from build123d import *

# Parameters (mm, degrees)
ESTRUSIONE_ESTRUSIONE1_DEPTH = 140
FORO_6_5_6_5_1_D             = 6.5
FORO_6_5_6_5_2_D             = 6.5
FORO_6_5_6_5_2_DEPTH         = 5
FORO_6_5_6_5_2_TIP           = 1.952797012
TAGLIO_ESTRUSIONE3_REACH     = 158.844
SCHIZZO10_R                  = 7
TAGLIO_ESTRUSIONE6_REACH     = 158.844
SMUSSO1_SIZE                 = 3
M3_TAPPED_HOLE1_D            = 2.5
M3_TAPPED_HOLE2_D            = 2.5


with BuildPart() as part:
    # Schizzo1 → Estrusione-Estrusione1 (new body)
    with BuildSketch(Plane.XY):
        Polygon((0, 0), (0, 50), (5, 50), (5, 5), (50, 5), (50, 0), align=None)
    extrude(amount=ESTRUSIONE_ESTRUSIONE1_DEPTH)

    # Foro Ø6.5 (6.5)-1 (through all)
    with Locations(Plane(origin=(0, 0, 0), x_dir=(-1, 0, 0), z_dir=(0, -1, 0))):
        with Locations((-17, -132), (-42, -132)):
            foro_6_5_6_5_1 = Hole(FORO_6_5_6_5_1_D / 2)

    # Foro Ø6.5 (6.5)-2
    with Locations(Plane.ZY):
        with Locations((132, 42), (132, 17)):
            Hole(FORO_6_5_6_5_2_D / 2, depth=FORO_6_5_6_5_2_DEPTH)
            with Locations((0, 0, -(FORO_6_5_6_5_2_DEPTH + FORO_6_5_6_5_2_TIP / 2))):  # 118° drill point
                Cone(0, FORO_6_5_6_5_2_D / 2, FORO_6_5_6_5_2_TIP, mode=Mode.SUBTRACT)

    # Specchia1: Foro Ø6.5 (6.5)-1 across plane
    add(foro_6_5_6_5_1.mirror(Plane.XY.offset(70)), mode=Mode.SUBTRACT)

    # Schizzo10 → Taglio-Estrusione3 (cut, up to next)
    with BuildSketch(Plane.ZY, mode=Mode.PRIVATE) as taglio_estrusione3_sk1:
        with Locations((80, 30)):
            Circle(SCHIZZO10_R)
    taglio_estrusione3_tool1 = extrude(taglio_estrusione3_sk1.sketch, amount=-TAGLIO_ESTRUSIONE3_REACH, mode=Mode.PRIVATE) & part.part
    add(taglio_estrusione3_tool1.solids().sort_by_distance((0, 30, 80))[0], mode=Mode.SUBTRACT)

    # Schizzo13 → Taglio-Estrusione6 (cut, up to next)
    with BuildSketch(Plane.ZY, mode=Mode.PRIVATE) as taglio_estrusione6_sk1:
        with BuildLine():
            Line((18, 43.306349186), (27, 43.306349186))
            ThreePointArc((27, 43.306349186), (28.75, 41.556349186), (27, 39.806349186))
            Line((27, 39.806349186), (18, 39.806349186))
            ThreePointArc((18, 39.806349186), (16.25, 41.556349186), (18, 43.306349186))
        make_face()
    taglio_estrusione6_tool1 = extrude(taglio_estrusione6_sk1.sketch, amount=-TAGLIO_ESTRUSIONE6_REACH, mode=Mode.PRIVATE) & part.part
    # Schizzo13 → Taglio-Estrusione6 (cut, up to next)
    with BuildSketch(Plane.ZY, mode=Mode.PRIVATE) as taglio_estrusione6_sk2:
        with BuildLine():
            Line((18, 8.693650814), (27, 8.693650814))
            ThreePointArc((27, 8.693650814), (28.75, 10.443650814), (27, 12.193650814))
            Line((27, 12.193650814), (18, 12.193650814))
            ThreePointArc((18, 12.193650814), (16.25, 10.443650814), (18, 8.693650814))
        make_face()
    taglio_estrusione6_tool2 = extrude(taglio_estrusione6_sk2.sketch, amount=-TAGLIO_ESTRUSIONE6_REACH, mode=Mode.PRIVATE) & part.part
    # Schizzo13 → Taglio-Estrusione6 (cut, up to next)
    with BuildSketch(Plane.ZY, mode=Mode.PRIVATE) as taglio_estrusione6_sk3:
        with BuildLine():
            Line((58, 43.306349186), (49, 43.306349186))
            ThreePointArc((49, 43.306349186), (47.25, 41.556349186), (49, 39.806349186))
            Line((49, 39.806349186), (58, 39.806349186))
            ThreePointArc((58, 39.806349186), (59.75, 41.556349186), (58, 43.306349186))
        make_face()
    taglio_estrusione6_tool3 = extrude(taglio_estrusione6_sk3.sketch, amount=-TAGLIO_ESTRUSIONE6_REACH, mode=Mode.PRIVATE) & part.part
    # Schizzo13 → Taglio-Estrusione6 (cut, up to next)
    with BuildSketch(Plane.ZY, mode=Mode.PRIVATE) as taglio_estrusione6_sk4:
        with BuildLine():
            Line((58, 8.693650814), (49, 8.693650814))
            ThreePointArc((49, 8.693650814), (47.25, 10.443650814), (49, 12.193650814))
            Line((49, 12.193650814), (58, 12.193650814))
            ThreePointArc((58, 12.193650814), (59.75, 10.443650814), (58, 8.693650814))
        make_face()
    taglio_estrusione6_tool4 = extrude(taglio_estrusione6_sk4.sketch, amount=-TAGLIO_ESTRUSIONE6_REACH, mode=Mode.PRIVATE) & part.part
    # Schizzo13 → Taglio-Estrusione6 (cut, up to next)
    with BuildSketch(Plane.ZY, mode=Mode.PRIVATE) as taglio_estrusione6_sk5:
        with BuildLine():
            Line((43, 14.75), (33, 14.75))
            ThreePointArc((33, 14.75), (21.75, 26), (33, 37.25))
            Line((33, 37.25), (43, 37.25))
            ThreePointArc((43, 37.25), (54.25, 26), (43, 14.75))
        make_face()
    taglio_estrusione6_tool5 = extrude(taglio_estrusione6_sk5.sketch, amount=-TAGLIO_ESTRUSIONE6_REACH, mode=Mode.PRIVATE) & part.part
    add(taglio_estrusione6_tool1.solids().sort_by_distance((0, 41.556349, 22.5))[0], mode=Mode.SUBTRACT)
    add(taglio_estrusione6_tool2.solids().sort_by_distance((0, 10.443651, 22.5))[0], mode=Mode.SUBTRACT)
    add(taglio_estrusione6_tool3.solids().sort_by_distance((0, 41.556349, 53.5))[0], mode=Mode.SUBTRACT)
    add(taglio_estrusione6_tool4.solids().sort_by_distance((0, 10.443651, 53.5))[0], mode=Mode.SUBTRACT)
    add(taglio_estrusione6_tool5.solids().sort_by_distance((0, 26, 38))[0], mode=Mode.SUBTRACT)

    # Smusso1
    smusso1_edges = [part.edges().sort_by_distance(p)[0] for p in [
        (2.5, 50, 140),
        (2.5, 50, 0),
        (50, 2.5, 140),
        (50, 2.5, 0),
    ]]
    chamfer(smusso1_edges, length=SMUSSO1_SIZE)

    # M3 Tapped Hole1 (through all)
    with Locations(Plane(origin=(0, 40, 70), x_dir=(0, 0, -1), z_dir=(-1, 0, 0))):
        with Locations((0, 0), (-20, 0), (-20, 20), (0, 20)):
            Hole(M3_TAPPED_HOLE1_D / 2)

    # M3 Tapped Hole2 (through all)
    with Locations(Plane(origin=(20, 0, 110), x_dir=(-1, 0, 0), z_dir=(0, -1, 0))):
        with Locations((0, 0), (-20, 0), (-20, 20), (0, 20)):
            Hole(M3_TAPPED_HOLE2_D / 2)


solid = part.part
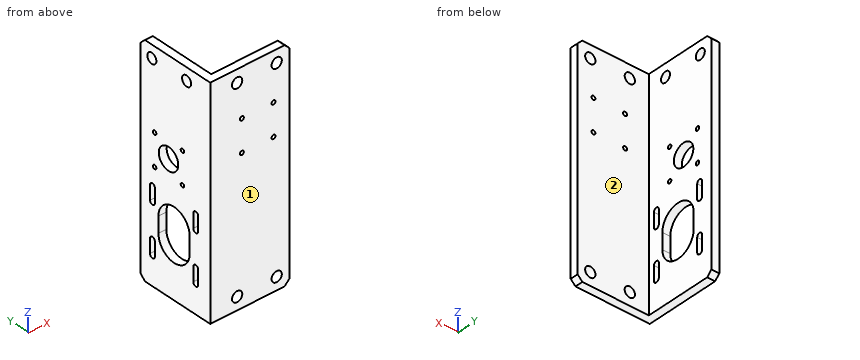
Could you check a few things on this model? Use its own coordinates, in mm. Face numbers are marked on the shaded views. A direction names the side the tool comes from. Give positions to 0.01 mm unless a question says otherwise; leave off trailing zeros. Order: outer loops, then holes, each group sorted by start corner. A loop starts at its lowest first (then second) coordinate and runs counter-clockwise, first axis right, second up.
1. I need wall thicknesses on L1, parallel to X at y = 3, z = 110; L2, parallel to Y at x = 3.2, z = 132. Which ranges of each line are inside material? Lowest first, please.
2. Suppose I cut it at D-D (z = 105.5). List the corners of the cut face in (x, y) for me.
3. For the marked faces 1 and 2, which set-ups out of +Z, -Z, +X, -X, +Y, -Y let a thin tool reach every point of the face, with its end or its side?
4. Suppose I cut it at B-B (z = 80). List the corners of the cut face in (x, y) for me, plus the area to 3 significant figures.
5. Suppose I cut it at C-C (y = 17). List the corners of the cut face in (x, z) for me, plus the area to 3 significant figures.
6. Will these pins go through, and if not, where does the flat tip stop? P1, Ø5, axis at y = 21, z = 83, coming from the +X side; P2, Ø4, axis at y = 20, z = 90, coming from the -X side; P3, Ø10.5, axis at x = 17, z = 8, coming from the +Y side.
7. Suppose I cut it at A-A (x = 17). List the corners of the cut face in (y, z) for me.
Solved:
1. L1: x = 0 to 18.75, 21.25 to 38.75, 41.25 to 50
1. L2: y = 0 to 13.75, 20.25 to 38.75, 45.25 to 50
2. outline: (0, 0) - (50, 0) - (50, 5) - (5, 5) - (5, 50) - (0, 50) - close
3. face 1: +Z, -Z, +X, -X, -Y
3. face 2: +Z, -Z, +X, +Y
4. outline: (0, 0) - (50, 0) - (50, 5) - (5, 5) - (5, 23) - (0, 23) - close; (0, 37) - (5, 37) - (5, 50) - (0, 50) - close
4. area: 405 mm2
5. outline: (0, 0) - (5, 0) - (5, 26.25) - (0, 26.25) - close; (0, 49.75) - (5, 49.75) - (5, 128.75) - (0, 128.75) - close; (0, 135.25) - (5, 135.25) - (5, 140) - (0, 140) - close
5. area: 550 mm2
6. P1: stops at x = 5
6. P2: stops at x = 0
6. P3: stops at y = 5
7. outline: (0, 0) - (5, 0) - (5, 4.75) - (0, 4.75) - close; (0, 11.25) - (5, 11.25) - (5, 128.75) - (0, 128.75) - close; (0, 135.25) - (5, 135.25) - (5, 140) - (0, 140) - close
